Could you check a few things on this drawing? It's one solid part, dimensions in mm from its lowest x, y, z. A direction names the side the tool comes from. Round coordinates to 2 decimals unless told otherwise and drop trailing zeros. Write each loop counter-clockwise with the first axis right and the second up, starting at its lowest first coordinate (ties: lowest second). Pieces come first, ordered by that corner, then holes. Notation, with made-up numbers: (60, 86) -> (87, 86) arc R18 ccw to (87, 99) -> close; hole circle Ø11 at (-29.5, 31). An arc over 180 degrees is marked (long way). Answer in a Markdown table with one row per item.
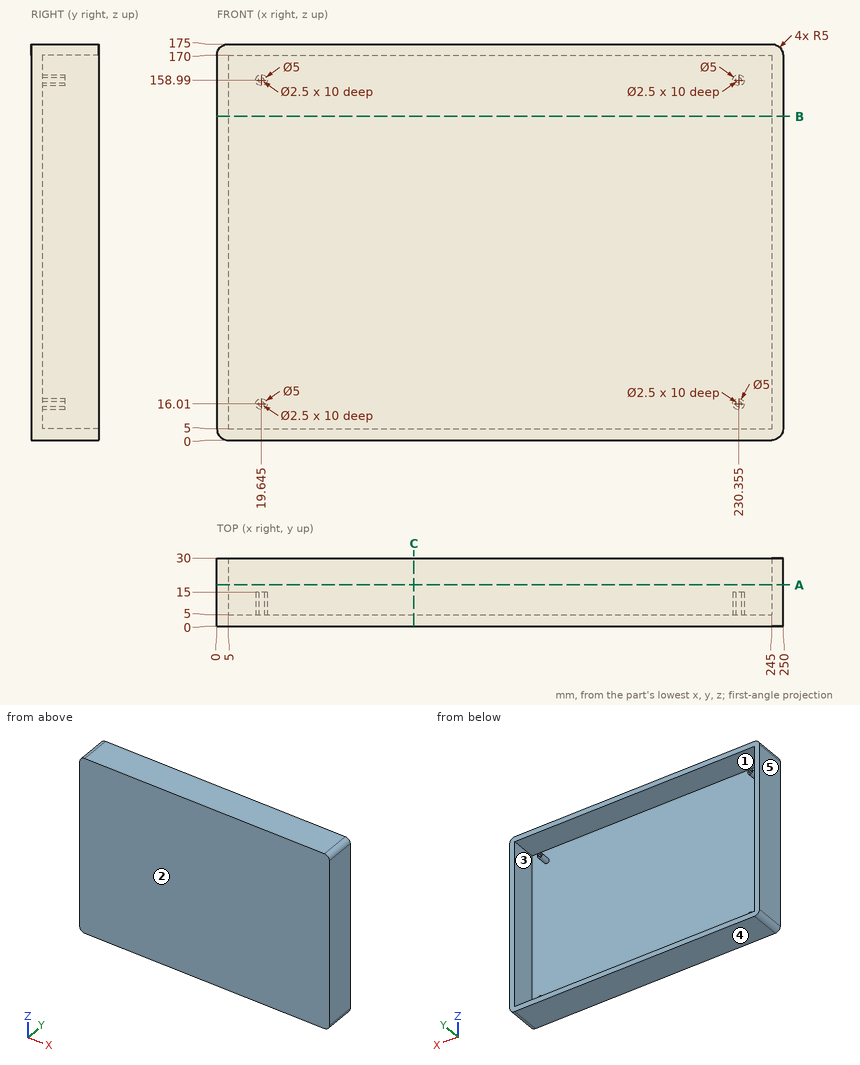
1) Imagine slicing it at A-A, the plane y = 18.25. Please give me the cut outline in (x, z).
Findings:
| item | result |
|---|---|
| outline | (0, 5) arc R5 ccw to (5, 0) -> (245, 0) arc R5 ccw to (250, 5) -> (250, 170) arc R5 ccw to (245, 175) -> (5, 175) arc R5 ccw to (0, 170) -> close; hole (5, 5) -> (245, 5) -> (245, 170) -> (5, 170) -> close |
2) Imagine slicing it at B-B, the plane z = 143. Please give me the cut outline in (x, y).
Findings:
| item | result |
|---|---|
| outline | (0, 0) -> (250, 0) -> (250, 30) -> (245, 30) -> (245, 5) -> (5, 5) -> (5, 30) -> (0, 30) -> close |
3) For the marked faces 1 and 2, which set-ups out of +Z, -Z, +X, -X, +Y, -Y let a thin tool reach every point of the face, with its end or its side?
Findings:
| item | result |
|---|---|
| face 1 | +Y |
| face 2 | +Z, -Z, +X, -X, -Y |
4) Please list where these lines run through material, in increasing order: line 1 (X direction, y = 8, z = 158.99) (3 decimals); line 2 (X direction, y = 17.25, z = 159.5); line 3 (Z direction, x = 48, y = 28).
Findings:
| item | result |
|---|---|
| line 1 | x = 0 to 5, 17.145 to 18.395, 20.895 to 22.145, 227.855 to 229.105, 231.605 to 232.855, 245 to 250 |
| line 2 | x = 0 to 5, 245 to 250 |
| line 3 | z = 0 to 5, 170 to 175 |
5) Thinking about a two-plate mould opening in X: for the marked faces 3, 4 and 5, which applies, +X half, -X half, draft (parallel to the pull), parting line (faces both ways), or undercut?
Findings:
| item | result |
|---|---|
| face 3 | undercut |
| face 4 | draft |
| face 5 | -X half |
6) For pin 1 (1.5 mm diameter, centred on x = 18.5, z = 159, fed in from +Y); pin 2 (1.2 mm diameter, centred on x = 19.5, z = 159.5, fed in from +Y), each with a flat end and sliding along its axis, tell me the tip position at first contact or that it passes through.
Findings:
| item | result |
|---|---|
| pin 1 | stops at y = 15 |
| pin 2 | stops at y = 5 |
7) Imagine slicing it at C-C, the plane x = 87. Please give me the cut outline in (y, z), plus the area to 4 significant figures.
Findings:
| item | result |
|---|---|
| outline | (0, 0) -> (30, 0) -> (30, 5) -> (5, 5) -> (5, 170) -> (30, 170) -> (30, 175) -> (0, 175) -> close |
| area | 1,125 mm^2 |
